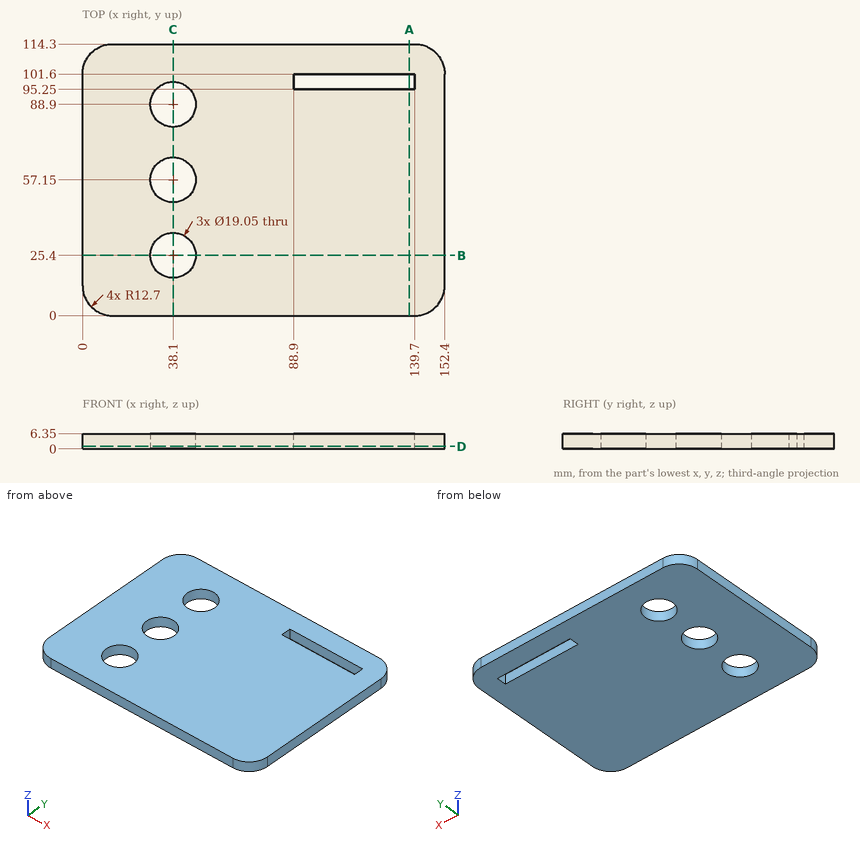
For this review, use the dimensioned drawing (mm, ordinates from the lowest corner) and the shaded views. Coordinates: 2 decimals unless noted, no trailing zeros. Order: outer loops, then holes, each group sorted by start corner. A loop starts at its lowest first (then second) coordinate and runs counter-clockwise, first axis right, second up. Notation, with made-up numbers: (-16.75, -2) -> (13.25, -2) arc R26 ccw to (13.25, 27) -> close; hole circle Ø8 at (-37, 31). An arc over 180 degrees is marked (long way). One line per item, written item: value. Start each with the question number.
Q1. For probe 1 along Y at (x, z) = (38.1, 4.25) (3 decimals); probe 2 along X at (y, z) = (25.5, 5.25); probe 3 along Y at (x, z) = (122, 5), list the stretches that pass through material, from the lowest coordinate up.
Q2. Take a section at C-C, the plane x = 38.1. State the section outline as (y, z) points (3 decimals), then the cut area to 3 significant figures.
Q3. Take a section at D-D, the plane z = 1. State the section outline as (x, y) points (3 decimals), then the cut area to 3 significant figures.
Q4. Insertion check: pin 1 Ø17 at (x, y) = (38.1, 25.4) entering from +Z. The pin has a flat end and moves straight along its axis. Give the tip position at first contact, or say it passes through.
Q5. Take a section at A-A, the plane x = 137.5. State the section outline as (y, z) points.
Q6. Take a section at B-B, the plane y = 25.4. State the section outline as (x, z) points (3 decimals).
Values follow:
1. probe 1: y = 0 to 15.875, 34.925 to 47.625, 66.675 to 79.375, 98.425 to 114.3
1. probe 2: x = 0 to 28.58, 47.62 to 152.4
1. probe 3: y = 0 to 95.25, 101.6 to 114.3
2. outline: (0, 0) -> (15.875, 0) -> (15.875, 6.35) -> (0, 6.35) -> close; (34.925, 0) -> (47.625, 0) -> (47.625, 6.35) -> (34.925, 6.35) -> close; (66.675, 0) -> (79.375, 0) -> (79.375, 6.35) -> (66.675, 6.35) -> close; (98.425, 0) -> (114.3, 0) -> (114.3, 6.35) -> (98.425, 6.35) -> close
2. area: 363 mm2
3. outline: (0, 12.7) arc R12.7 ccw to (12.7, 0) -> (139.7, 0) arc R12.7 ccw to (152.4, 12.7) -> (152.4, 101.6) arc R12.7 ccw to (139.7, 114.3) -> (12.7, 114.3) arc R12.7 ccw to (0, 101.6) -> close; hole circle Ø19.05 at (38.1, 25.4); hole circle Ø19.05 at (38.1, 57.15); hole circle Ø19.05 at (38.1, 88.9); hole (88.9, 95.25) -> (139.7, 95.25) -> (139.7, 101.6) -> (88.9, 101.6) -> close
3. area: 16,100 mm2
4. pin 1: passes through
5. outline: (0, 0) -> (95.25, 0) -> (95.25, 6.35) -> (0, 6.35) -> close; (101.6, 0) -> (114.3, 0) -> (114.3, 6.35) -> (101.6, 6.35) -> close
6. outline: (0, 0) -> (28.575, 0) -> (28.575, 6.35) -> (0, 6.35) -> close; (47.625, 0) -> (152.4, 0) -> (152.4, 6.35) -> (47.625, 6.35) -> close
